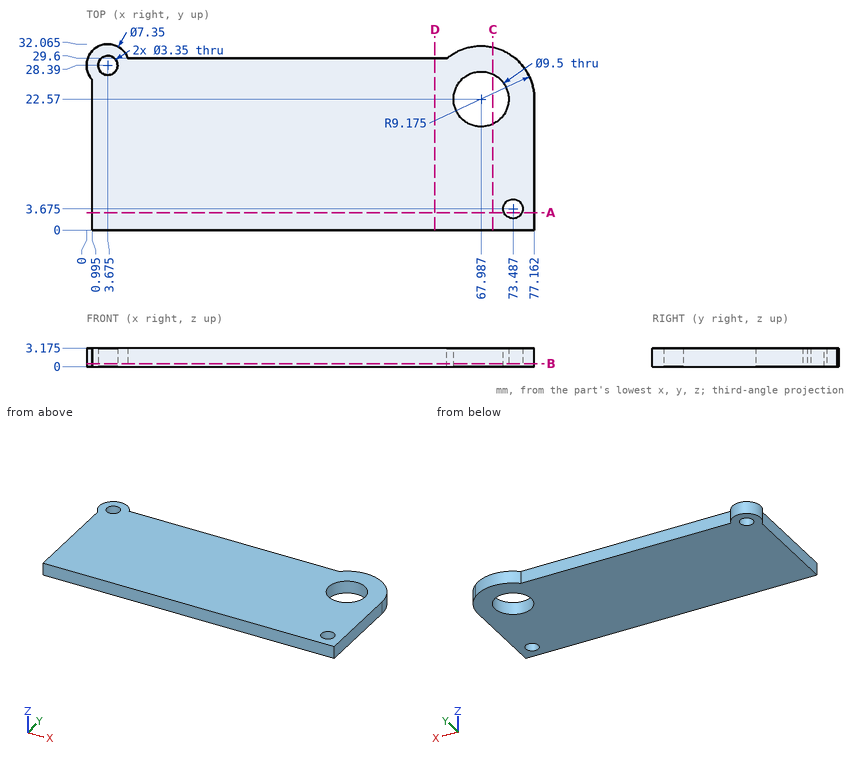
Verification items for this drawing (mm, ordinates from the low corner). Coordinates: 2 decimals unless noted, no trailing zeros. Write each loop counter-clockwise with the first axis right and the second up, starting at its lowest first coordinate (ties: lowest second). Pieces come first, ordered by that corner, then holes. Notation, with made-up numbers: M 31.5,-34.75 L 39.5,-34.75 A22 cw 39.5,-6.75 Z; hole C -22.75,-25 d8. An arc over 180 degrees is marked long. One line per item, written item: value. Start each with the question number.
(1) Scan lines: line 1 along X through (y, z) = (22.5, 2.9) (3 decimals); line 2 along Y through (x, z) = (68, 1.95) (3 decimals); line 3 along Y through (x, z) = (47.5, 0.9). Record each from-to range of solid material in increasing order. Write a range as [from, to].
(2) Sectioned sample at C-C, the plane x = 70. Enter the section's corners in (y, z) (3 decimals), and give its area (3 significant figures).
(3) Sectioned sample at D-D, the plane x = 60. Enter the section's corners in (y, z) (3 decimals).
(4) Sectioned sample at B-B, the plane z = 0.5. Enter the section's corners in (x, y) (3 decimals), and give its area (3 significant figures).
(5) Sectioned sample at A-A, the plane y = 3. Enter the section's corners in (x, z) (3 decimals).
Filled sheet:
1. line 1: [0.995, 63.238], [72.736, 77.162]
1. line 2: [0, 17.82], [27.32, 31.745]
1. line 3: [0, 29.6]
2. outline: M 0,0 L 18.268,0 L 18.268,3.175 L 0,3.175 Z; M 26.872,0 L 31.521,0 L 31.521,3.175 L 26.872,3.175 Z
2. area: 72.8 mm²
3. outline: M 0,0 L 29.6,0 L 29.6,3.175 L 0,3.175 Z
4. outline: M 0.995,0 L 77.162,0 L 77.162,22.57 A9.175 ccw 62.091,29.6 L 7.145,29.6 A3.675 ccw long 0.995,25.875 Z; hole C 3.675,28.39 d3.35; hole C 67.987,22.57 d9.5; hole C 73.487,3.675 d3.35
4. area: 2,190 mm²
5. outline: M 0.995,0 L 71.954,0 L 71.954,3.175 L 0.995,3.175 Z; M 75.02,0 L 77.162,0 L 77.162,3.175 L 75.02,3.175 Z
